Here's how the part is built. I have some questions about the finished solid (model axes, mm). Coordinates: 2 decimals unless noted, no trailing zeros. Order: outer loops, then holes, each group sorted by start corner. A loop starts at its lowest first (then second) coordinate and runs counter-clockwise, first axis right, second up. Notation, with made-up numbers: (57.25, 82) - (61.25, 82) arc R22 ccw to (61.25, 102) - close; hole circle Ø10 at (-33, 77.25). An arc over 180 degrees is marked (long way). Use CSV: the item, a comma, the result in double quotes. Start each with the question number.
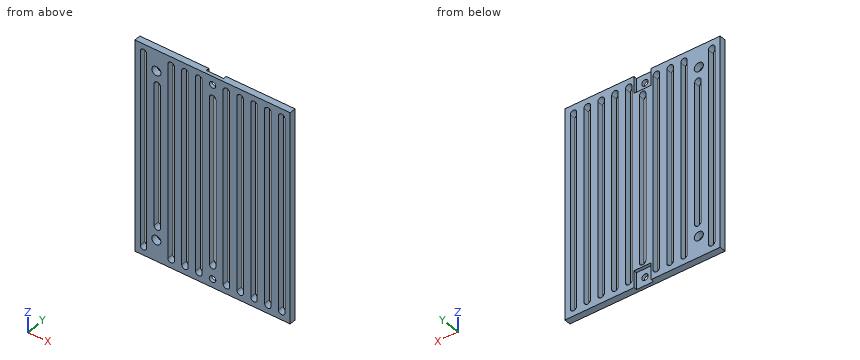
Autodesk Inventor part; units mm, degrees
ref_plane "YZ Plane" through (0, 0, 0) normal (1, 0, 0) x (0, 1, 0)
ref_plane "XZ Plane" through (0, 0, 0) normal (0, 1, 0) x (-1, 0, 0)
ref_plane "XY Plane" through (0, 0, 0) normal (0, 0, 1) x (1, 0, 0)
sketch "Sketch1" plane through (0, 0, 0) normal (0, 1, 0) x (-1, 0, 0)
  line L0 (0, 0) -> (-72.5, 0)
  line L1 (-72.5, 0) -> (-72.5, -100)
  line L2 (-72.5, -100) -> (0, -100)
  line L3 (0, -100) -> (0, 0)
  dimension "d0" = 72.5
  dimension "d1" = 100
extrude "Extrusion1" add sketch "Sketch1" along normal blind 3
sketch "Sketch7" plane through (0, 3, 0) normal (0, 1, 0) x (1, 0, 0)
  line L0 (72.5, 100) -> (0, 100)
  line L1 (0, 0) -> (72.5, 0)
  line L2 (72.5, 0) -> (72.5, 100)
  line L3 (72.5, 100) -> (0, 100)
  line L4 (0, 100) -> (0, 0)
  line L5 (0, 0) -> (0, 9.525)
  line L6 (0, 0) -> (10, 0)
  line L7 (10, 0) -> (10, 10)
  line L8 (10, 10) -> (0, 10)
  line L9 (0, 10) -> (0, 0)
  line L10 (0, 100) -> (10, 100)
  line L11 (10, 100) -> (10, 90)
  line L12 (10, 90) -> (0, 90)
  line L13 (0, 90) -> (0, 100)
  line L14 (72.5, 100) -> (62.5, 100)
  line L15 (62.5, 100) -> (62.5, 90)
  line L16 (62.5, 90) -> (72.5, 90)
  line L17 (72.5, 90) -> (72.5, 100)
  circle A0 centre (95, 95) radius 1.5
  line L18 (72.5, 0) -> (62.5, 0)
  line L19 (62.5, 0) -> (62.5, 10)
  line L20 (62.5, 10) -> (72.5, 10)
  line L21 (72.5, 10) -> (72.5, 0)
  circle A1 centre (95, 5) radius 1.5
  circle A2 centre (10, 90) radius 2.125
  circle A3 centre (10, 10) radius 2.125
  point P0 (41.25, 100)
  dimension "d36" = 10
  dimension "d37" = 10
  dimension "d39" = 10
  dimension "d40" = 10
  dimension "d42" = 10
  dimension "d43" = 10
  dimension "d44" = 3
  dimension "d45" = 10
  dimension "d46" = 10
  dimension "d47" = 3
  dimension "d181" = 4.25
  dimension "d182" = 4.25
extrude "Extrusion7" cut sketch "Sketch7" against normal blind 3 contours A2 L12 L11 | L11 L12 A2 | A3 L7 L8 | L8 L7 A3 | A0 | A1
sketch "Sketch11" plane through (0, 3, 0) normal (0, 1, 0) x (1, 0, 0)
  point P0 (0, 0)
sketch "Sketch13" plane through (0, 3, 0) normal (0, 1, 0) x (1, 0, 0)
  line L0 (0, 0) -> (72.5, 0)
  line L1 (36.25, 0) -> (36.25, 8)
  line L2 (36.25, 8) -> (32.25, 8)
  line L3 (32.25, 8) -> (32.25, 0)
  line L4 (36.25, 0) -> (32.25, 0)
  line L5 (36.25, 0) -> (40.25, 0)
  line L6 (40.25, 0) -> (40.25, 8)
  line L7 (40.25, 8) -> (36.25, 8)
  line L8 (72.5, 100) -> (0, 100)
  line L9 (36.25, 100) -> (32.25, 100)
  line L10 (32.25, 100) -> (32.25, 92)
  line L11 (32.25, 92) -> (40.25, 92)
  line L12 (40.25, 92) -> (40.25, 100)
  line L13 (40.25, 100) -> (36.25, 100)
  line L14 (72.5, 0) -> (72.5, 100)
  dimension "d190" = 8
  dimension "d191" = 4
  dimension "d192" = 4
  dimension "d193" = 8
extrude "Extrusion11" cut sketch "Sketch13" against normal blind 1.5
sketch "Sketch14" plane through (0, 1.5, 0) normal (0, 1, 0) x (1, 0, 0)
  line L0 (0, 0) -> (72.5, 0)
  line L1 (40.25, 8) -> (32.25, 8)
  line L2 (32.25, 8) -> (32.25, 0)
  line L3 (32.25, 0) -> (40.25, 0)
  line L4 (40.25, 0) -> (40.25, 8)
  line L5 (72.5, 100) -> (0, 100)
  line L6 (40.25, 100) -> (32.25, 100)
  line L7 (32.25, 100) -> (32.25, 92)
  line L8 (32.25, 92) -> (40.25, 92)
  line L9 (40.25, 92) -> (40.25, 100)
  circle A0 centre (36.25, 4) radius 1.5
  circle A1 centre (36.25, 96) radius 1.5
  point P0 (72.5, 46)
  point P1 (64.5, 54)
  dimension "d199" = 8
  dimension "d200" = 8
  dimension "d201" = 3
  dimension "d202" = 3
extrude "Extrusion12" cut sketch "Sketch14" against normal blind 1.5 contours A0 | A1
sketch "Sketch15" plane through (0, 3, 0) normal (0, 1, 0) x (1, 0, 0)
  circle A0 centre (36.25, 4) radius 1.5
  line L0 (0, 100) -> (0, 0)
  circle A1 centre (36.25, 96) radius 1.5
  line L1 (32.25, 8) -> (40.25, 8)
  arc A2 (2.5, 4) -> (5.5, 4) centre (4, 4) ccw
  arc A3 (15.4, 4) -> (18.4, 4) centre (16.9, 4) ccw
  arc A4 (21.85, 4) -> (24.85, 4) centre (23.35, 4) ccw
  arc A5 (28.3, 4) -> (31.3, 4) centre (29.8, 4) ccw
  arc A6 (41.2, 4) -> (44.2, 4) centre (42.7, 4) ccw
  arc A7 (47.65, 4) -> (50.65, 4) centre (49.15, 4) ccw
  arc A8 (54.1, 4) -> (57.1, 4) centre (55.6, 4) ccw
  arc A9 (60.55, 4) -> (63.55, 4) centre (62.05, 4) ccw
  arc A10 (67, 4) -> (70, 4) centre (68.5, 4) ccw
  arc A11 (70, 96) -> (67, 96) centre (68.5, 96) ccw
  arc A12 (63.55, 96) -> (60.55, 96) centre (62.05, 96) ccw
  arc A13 (57.1, 96) -> (54.1, 96) centre (55.6, 96) ccw
  arc A14 (50.65, 96) -> (47.65, 96) centre (49.15, 96) ccw
  arc A15 (44.2, 96) -> (41.2, 96) centre (42.7, 96) ccw
  arc A16 (31.3, 96) -> (28.3, 96) centre (29.8, 96) ccw
  arc A17 (24.85, 96) -> (21.85, 96) centre (23.35, 96) ccw
  arc A18 (18.4, 96) -> (15.4, 96) centre (16.9, 96) ccw
  arc A19 (5.5, 96) -> (2.5, 96) centre (4, 96) ccw
  circle A20 centre (10, 90) radius 2.125
  line L2 (10, 90) -> (10.45, 90)
  line L3 (10.45, 90) -> (10.45, 83.55)
  arc A21 (11.95, 83.55) -> (8.95, 83.55) centre (10.45, 83.55) ccw
  circle A22 centre (10, 10) radius 2.125
  line L4 (10, 10) -> (10.45, 10)
  line L5 (10.45, 10) -> (10.45, 16.45)
  arc A23 (8.95, 16.45) -> (11.95, 16.45) centre (10.45, 16.45) ccw
  line L6 (5.5, 4) -> (5.5, 96)
  line L7 (2.5, 96) -> (2.5, 4)
  line L8 (8.95, 16.45) -> (8.95, 83.55)
  line L9 (11.95, 83.55) -> (11.95, 16.45)
  line L10 (15.4, 4) -> (15.4, 96)
  line L11 (18.4, 96) -> (18.4, 4)
  line L12 (21.85, 96) -> (21.85, 4)
  line L13 (24.85, 4) -> (24.85, 96)
  line L14 (28.3, 96) -> (28.3, 4)
  line L15 (31.3, 4) -> (31.3, 96)
  line L16 (41.2, 96) -> (41.2, 4)
  line L17 (44.2, 4) -> (44.2, 96)
  line L18 (47.65, 96) -> (47.65, 4)
  line L19 (50.65, 4) -> (50.65, 96)
  line L20 (54.1, 96) -> (54.1, 4)
  line L21 (57.1, 4) -> (57.1, 96)
  line L22 (60.55, 96) -> (60.55, 4)
  line L23 (63.55, 4) -> (63.55, 96)
  line L24 (67, 43.55) -> (67, 4)
  line L25 (70, 4) -> (70, 43.55)
  line L26 (67, 56.45) -> (67, 96)
  line L27 (70, 96) -> (70, 56.45)
  line L28 (36.25, 4) -> (36.25, 10.45)
  arc A24 (34.75, 10.45) -> (37.75, 10.45) centre (36.25, 10.45) ccw
  line L29 (36.25, 96) -> (36.25, 89.55)
  arc A25 (37.75, 89.55) -> (34.75, 89.55) centre (36.25, 89.55) ccw
  line L30 (34.75, 10.45) -> (34.75, 89.55)
  line L31 (37.75, 89.55) -> (37.75, 10.45)
  line L32 (67, 56.45) -> (67, 43.55)
  line L33 (70, 43.55) -> (70, 56.45)
  dimension "d216" = 3
  dimension "d217" = 3
  dimension "d218" = 3
  dimension "d219" = 3
  dimension "d220" = 3
  dimension "d221" = 3
  dimension "d225" = 3
  dimension "d226" = 3
  dimension "d227" = 3
  dimension "d228" = 3
  dimension "d229" = 3
  dimension "d230" = 3
  dimension "d231" = 3
  dimension "d232" = 3
  dimension "d233" = 3
  dimension "d234" = 6.45
  dimension "d235" = 3
  dimension "d236" = 6.45
  dimension "d237" = 3
  dimension "d242" = 6.45
  dimension "d243" = 3
  dimension "d244" = 6.45
  dimension "d245" = 3
extrude "Extrusion13" cut sketch "Sketch15" against normal blind 3 contours A24 L30 A25 L31 | L7 A19 L6 A2 | L10 A18 L11 A3 | L12 A17 L13 A4 | L14 A16 L15 A5 | L16 A15 L17 A6 | L18 A14 L19 A7 | L20 A13 L21 A8 | L22 A12 L23 A9 | L24 L32 L26 A11 L27 L33 L25 A10 | A21 L9 A23 L8
sketch "Sketch16" plane through (0, 3, 0) normal (0, 1, 0) x (1, 0, 0)
  point P0 (0, 0)
properties part number "Tray"
Item 1: For pin 1 Ø5 at (x, z) = (36.25, -4) entering from +Y, with a flat end and sliding along its axis, tell me the tip position at first contact or that it passes through.
Item 2: Suppose I cut it at A-A on x = 55.6. Write out the boundary of the cut face in (y, z).
Item 3: Suppose I cut it at B-B on x = 10. Write out the boundary of the cut face in (y, z) (3 decimals).
Item 4: Please list where these lines run through material, in increasing order: line 1 along Z through (x, y) = (36.25, 1); line 2 along Z through (x, y) = (10, 2.1) (3 decimals); line 3 along Z through (x, y) = (24.5, 1.8). Write a range as from..to.
Item 5: Suppose I cut it at C-C on z = -31.5. State how many separate pieces and enclosed holes the cut face has, then the cut area to 4 significant figures.
Here are the results:
1,pin 1,"y = 1.5"
2,outline,"(0, -100) - (3, -100) - (3, -97.5) - (0, -97.5) - close; (0, -2.5) - (3, -2.5) - (3, 0) - (0, 0) - close"
3,outline,"(0, -100) - (3, -100) - (3, -92.125) - (0, -92.125) - close; (0, -87.875) - (3, -87.875) - (3, -84.981) - (0, -84.981) - close; (0, -15.019) - (3, -15.019) - (3, -12.125) - (0, -12.125) - close; (0, -7.875) - (3, -7.875) - (3, 0) - (0, 0) - close"
4,line 1,"-100..-97.5, -94.5..-91.05, -8.95..-5.5, -2.5..0"
4,line 2,"-100..-92.125, -87.875..-84.981, -15.019..-12.125, -7.875..0"
4,line 3,"-100..-96.96, -3.04..0"
5,separate pieces,"12"
5,enclosed holes,"0"
5,area,"118.5 mm^2"
